The listing builds one solid part. Answer for the finished solid, in the listing's coordinates (mm). A direction names the side the tool comes from. Round coordinates to 2 decimals unless told otherwise and drop trailing zeros. Write each loop counter-clockwise with the first axis right and the second up, starting at its lowest first coordinate (ties: lowest second). Pieces come first, ordered by that corner, then holes. Notation, with made-up numbers: M 4.5,-37 L 11.5,-37 A13 cw 11.5,-32 Z; hole C 23,61 d5. An arc over 180 degrees is marked long. One line per item, written item: value. Start each with the question number.
(1) For a pull along X with two mould halves and no side action, classify faces 1 (the flat face through (348.001, 29.58, 195.145)), 2 (the flat face through (243.5, 29.6, -15.3)), 3 (the flat face through (-354.336, 29.58, 279.632)), 4 (the flat face through (-240.481, 29.58, -17.043)) as released by +X, released by -X, zero draft, split by the parting line, or undercut.
(2) Given P1, Ø1, axis at y = 27, z = -269.5, coming from the -X side; P2, Ø10, axis at x = -118.5, y = 50, coming from the +Z side; P3, Ø11, axis at x = 0, y = 45, coming from the +Z side, each flat-ended and moving along its own axis, determine where each tip first touches the part or whether it passes through.
(3) Section B-B (x = -89) is taken. Determine the outline of the cut face in (y, z), plus the area to 3 significant figures.
(4) Section D-D (z = -57) is taken. Determine the outline of the cut face in (x, y).
(5) Consider probe 1 along X at (y, z) = (29, -139.5); probe 2 along X at (y, z) = (52, 62); probe 3 along X at (y, z) = (39, -360). Determine where each line is inside the solid, lowest interval first.
(6) For faces 5 (the flat face through (1, 30, -565)), 6 (the flat face through (344.819, 29.58, 204.855)), 7 (the flat face through (488.85, 29.58, 283.29)), 8 (the flat face through (-231.7, 29.58, 248.68)), 9 (the flat face through (-331.703, 29.58, 75.473)), determine the directions among +Z, -Z, +X, -X, +Y, -Y from which every point of the face is accessible in a straight line to the end or side of a thin tool.
(7) Section C-C (y = 32) is taken. State how many separate pieces and enclosed holes the cut face has, plus the area to 3 significant figures.
(8) Section A-A (z = -342.5) is taken. Determine the outline of the cut face in (x, y), plus the area to 3 significant figures.
```python
from build123d import *

# Parameters (mm, degrees)
CROQUIS1_W              = 90
CROQUIS1_H              = 119.019237886
CROQUIS1_W_2            = 10
CROQUIS1_H_2            = 150
SALIENTE_EXTRUIR1_DEPTH = 60


with BuildPart() as part:
    # Croquis1 → Saliente-Extruir1 (new body)
    with BuildSketch(Plane(origin=(0, 0, 0), x_dir=(1, 0, 0), z_dir=(0, 1, 0))):
        Polygon((-213.95825623, -279.413429511), (0, -155.884572681), (213.95825623, -279.413429511), (248.95825623, -218.791651246), (456.804353138, -338.791651246), (521.804353138, -226.208348754), (313.95825623, -106.208348754), (348.95825623, -45.586570489), (135, 77.942286341), (135, 325), (65, 325), (65, 565), (-65, 565), (-65, 325), (-135, 325), (-135, 77.942286341), (-348.95825623, -45.586570489), (-313.95825623, -106.208348754), (-521.804353138, -226.208348754), (-456.804353138, -338.791651246), (-248.95825623, -218.791651246), align=None)
        Polygon((278.95825623, -166.830127019), (283.95825623, -158.169872981), (348.910161514, -195.669872981), (413.862066798, -233.169872981), (408.862066798, -241.830127019), (343.910161514, -204.330127019), align=None, mode=Mode.SUBTRACT)
        Polygon((-408.862066798, -241.830127019), (-413.862066798, -233.169872981), (-283.95825623, -158.169872981), (-278.95825623, -166.830127019), align=None, mode=Mode.SUBTRACT)
        Polygon((-122.942286341, -19.019237886), (-77.942286341, -96.961524227), (-181.015969889, -156.47114317), (-226.015969889, -78.52885683), align=None, mode=Mode.SUBTRACT)
        Polygon((181.015969889, -156.47114317), (77.942286341, -96.961524227), (122.942286341, -19.019237886), (226.015969889, -78.52885683), align=None, mode=Mode.SUBTRACT)
        Polygon((0, -51.961524227), (-45, 25.980762114), (45, 25.980762114), align=None, mode=Mode.SUBTRACT)
        with Locations((0, 175.490381057)):
            Rectangle(CROQUIS1_W, CROQUIS1_H, mode=Mode.SUBTRACT)
        with Locations((0, 400)):
            Rectangle(CROQUIS1_W_2, CROQUIS1_H_2, mode=Mode.SUBTRACT)
    extrude(amount=SALIENTE_EXTRUIR1_DEPTH)


solid = part.part
```
Recorded:
1. face 1: undercut
1. face 2: released by +X
1. face 3: undercut
1. face 4: released by -X
2. P1: stops at x = -135
2. P2: stops at z = 227.19
2. P3: stops at z = 159.06
3. outline: M 0,-325 L 60,-325 L 60,77.81 L 0,77.81 Z; M 0,103.35 L 60,103.35 L 60,207.27 L 0,207.27 Z
3. area: 30,400 mm2
4. outline: M -171.27,0 L 171.27,0 L 171.27,60 L -171.27,60 Z
5. probe 1: x = -135 to -45, 45 to 135
5. probe 2: x = -339.48 to -197.39, -98.13 to 98.13, 197.39 to 339.48
5. probe 3: x = -65 to -5, 5 to 65
6. face 5: -Z, +X, -X, +Y, -Y
6. face 6: +Y, -Y
6. face 7: +Z, +X, +Y, -Y
6. face 8: +Z, +Y, -Y
6. face 9: -X, +Y, -Y
7. separate pieces: 1
7. enclosed holes: 7
7. area: 285,000 mm2
8. outline: M -65,0 L -5,0 L -5,60 L -65,60 Z; M 5,0 L 65,0 L 65,60 L 5,60 Z
8. area: 7,200 mm2
